Read the model definition and answer for the solid it produces. Units are mm, in the model's axes. A direction names the side the tool comes from. Coordinates: 2 decimals unless noted, no trailing zeros. Write each loop counter-clockwise with the first axis right and the second up, starting at its lowest first coordinate (ties: lowest second). Pieces come first, ordered by that corner, then holes.
(1) Given pin 1 (15.5 mm diameter, centred on y = -40.5, z = 2, fed in from +X); pin 2 (12 mm diameter, centred on y = -72, z = 9.5, fed in from -X); pin 3 (5 mm diameter, centred on x = 7.5, z = 11.5, fed in from +Y); pin 4 (5 mm diameter, centred on x = -1, y = -34, fed in from -Z), each flat-ended and moving along its own axis, determine where each tip first touches the part or whether it passes through.
(2) Section B-B on y = -108.5 is taken. Write down the section's boundary in (x, z), then the cut area to 3 significant figures.
(3) Find the intervals of material crossed by probe 1 along Z at (x, y) = (0, -99.9); probe 2 along X at (y, z) = (-4, 0); probe 3 along Z at (x, y) = (0, -41.5) (3 decimals), in increasing order.
(4) Section A-A on y = -68.5 is taken. Write down the section's boundary in (x, z) (3 decimals), then the cut area to 3 significant figures.
(5) Which of the six approach directions +Z, -Z, +X, -X, +Y, -Y give full straight-line access (tool end or side, diameter ignored) to faces 1 (the flat face through (-1, -97.5, 10)), 2 (the flat face through (10, -55, -1)), 3 (the cylindrical face through (-1.73, -100.01, -7.81)), 4 (the flat face through (5.2, -12, -0.1)), 5 (the flat face through (0, -97.5, -13))?
(6) The mould has two halves that part along Z. Classify faces 6 (the flat face through (-1, -13.5, 10)), 7 (the cylindrical face through (-1.73, -10.99, 7.81)), 8 (the cylindrical face through (7.768, -114.14, 12.184)): +Z half, -Z half, draft (parallel to the pull), parting line (faces both ways), or undercut.
from build123d import *

# Parameters (mm, degrees)
SKETCH_R        = 14.95
PAD001_DEPTH    = 124
SKETCH001_R     = 11
POCKET_DEPTH    = 10
SKETCH021_R     = 8
POCKET007_DEPTH = 2
SKETCH002_R     = 5.005
POCKET001_DEPTH = 114.001
SKETCH003_R     = 11
POCKET002_DEPTH = 23
SKETCH022_R     = 8
POCKET008_DEPTH = 2
SKETCH004_W     = 30.9
SKETCH004_H     = 30.9
POCKET003_DEPTH = 84
SKETCH015_R     = 15.45
SKETCH015_R_2   = 14.45
POCKET005_DEPTH = 20


with BuildPart() as part:
    # Sketch → Pad001 (new body)
    with BuildSketch(Plane.XZ):
        Circle(SKETCH_R)
    extrude(amount=PAD001_DEPTH)

    # Sketch001 (on Face2 of Pad001) → Pocket (cut)
    with BuildSketch(Plane(origin=(0, 0, 0), x_dir=(1, 0, 0), z_dir=(0, 1, 0))):
        Circle(SKETCH001_R)
    extrude(amount=-POCKET_DEPTH, mode=Mode.SUBTRACT)

    # Sketch021 (on Face5 of Pocket) → Pocket007 (cut)
    with BuildSketch(Plane(origin=(0, -10, 0), x_dir=(1, 0, 0), z_dir=(0, 1, 0))):
        Circle(SKETCH021_R)
    extrude(amount=-POCKET007_DEPTH, mode=Mode.SUBTRACT)

    # Sketch002 (on Face5 of Pocket) → Pocket001 (cut, through all)
    with BuildSketch(Plane(origin=(0, -10, 0), x_dir=(1, 0, 0), z_dir=(0, 1, 0))):
        Circle(SKETCH002_R)
    extrude(amount=-POCKET001_DEPTH, mode=Mode.SUBTRACT)

    # Sketch003 (on Face3 of Pocket001) → Pocket002 (cut)
    with BuildSketch(Plane.XZ.offset(124)):
        Circle(SKETCH003_R)
    extrude(amount=-POCKET002_DEPTH, mode=Mode.SUBTRACT)

    # Sketch022 (on Face7 of Pocket002) → Pocket008 (cut)
    with BuildSketch(Plane.XZ.offset(101)):
        Circle(SKETCH022_R)
    extrude(amount=-POCKET008_DEPTH, mode=Mode.SUBTRACT)

    # Sketch004 → Pocket003 (cut)
    with BuildSketch(Plane.XZ.offset(13.5)):
        Rectangle(SKETCH004_W, SKETCH004_H)
        Polygon((-9.292893, -12.5), (9.292893, -12.5), (10, -11.792893), (10, 8.5), (-10, 8.5), (-10, -11.792893), align=None, mode=Mode.SUBTRACT)
    extrude(amount=POCKET003_DEPTH, mode=Mode.SUBTRACT)

    # Sketch015 (on Face6 of Pocket003) → Pocket005 (cut)
    with BuildSketch(Plane.XZ.offset(124)):
        Circle(SKETCH015_R)
        Circle(SKETCH015_R_2, mode=Mode.SUBTRACT)
    extrude(amount=-POCKET005_DEPTH, mode=Mode.SUBTRACT)


solid = part.part
Response:
1. pin 1: stops at x = 10
1. pin 2: stops at x = -10
1. pin 3: stops at y = 0
1. pin 4: stops at z = -12.5
2. outline: circle Ø28.9 at (0, 0); hole circle Ø22 at (0, 0)
2. area: 276 mm2
3. probe 1: z = -14.95 to -8, 8 to 14.95
3. probe 2: x = -14.95 to -11, 11 to 14.95
3. probe 3: z = -12.5 to -5.005, 5.005 to 8.5
4. outline: (-10, -11.113) arc R14.95 ccw to (-8.201, -12.5) - (8.201, -12.5) arc R14.95 ccw to (10, -11.113) - (10, 8.5) - (-10, 8.5) - close; hole circle Ø10.01 at (0, 0)
4. area: 339 mm2
5. face 1: +Z
5. face 2: +Z, -Z, +X
5. face 3: -Y
5. face 4: +Y
5. face 5: -Z, +X, -X
6. face 6: draft
6. face 7: undercut
6. face 8: parting line
